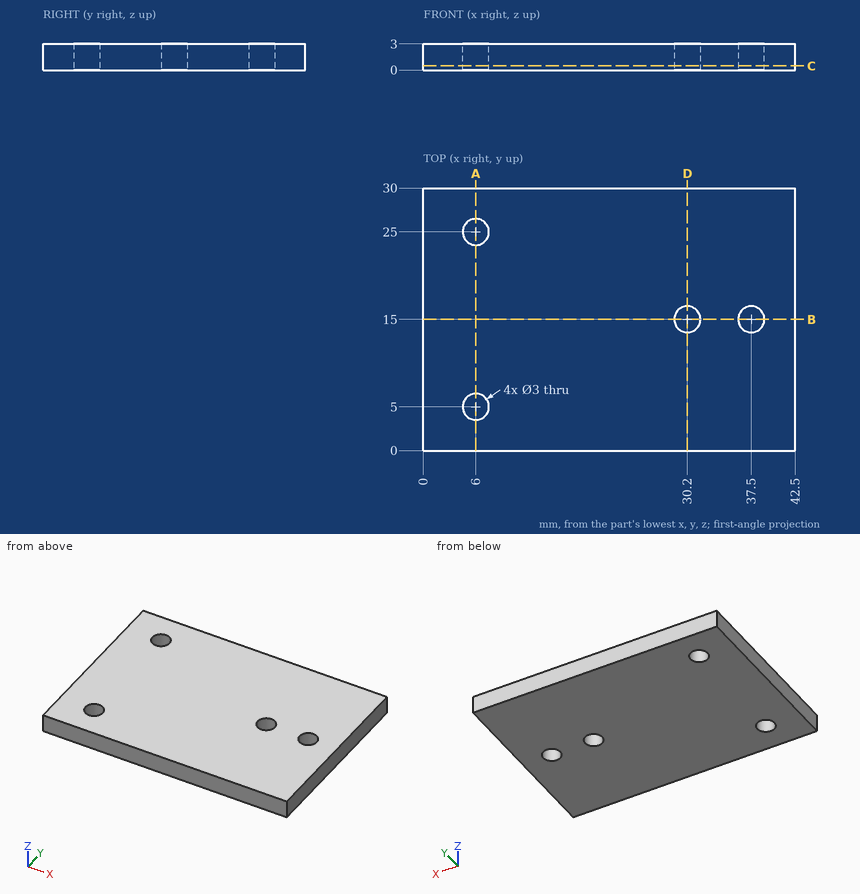
Geometry check sheet. Reference: drawing and pictorial views, mm from the part's lowest x, y, z. Round coordinates to 2 decimals unless told otherwise and drop trailing zeros. Write each loop counter-clockwise with the first axis right and the second up, starting at its lowest first coordinate (ties: lowest second). Pieces come first, ordered by that corner, then holes.
1. Gauge pin test, flat end, axial feed: P1, Ø1.8, axis at x = 6, y = 5, coming from the -Z side. Record the tip position at first contact, or that the pin passes through.
2. Section check D-D on x = 30.2. Enter the section's corners in (y, z), plus the area to 3 significant figures.
3. Section check B-B on y = 15. Enter the section's corners in (x, z).
4. Section check A-A on x = 6. Enter the section's corners in (y, z).
5. Scan lines: L1, parallel to Y at x = 6, z = 1.6; L2, parallel to Y at x = 30.2, z = 2.1; L3, parallel to X at y = 5, z = 1.75. Record each from-to range of solid material in increasing order.
6. Section check C-C on z = 0.5. Enter the section's corners in (x, y).
Answer:
1. P1: passes through
2. outline: (0, 0) - (13.5, 0) - (13.5, 3) - (0, 3) - close; (16.5, 0) - (30, 0) - (30, 3) - (16.5, 3) - close
2. area: 81.0 mm2
3. outline: (0, 0) - (28.7, 0) - (28.7, 3) - (0, 3) - close; (31.7, 0) - (36, 0) - (36, 3) - (31.7, 3) - close; (39, 0) - (42.5, 0) - (42.5, 3) - (39, 3) - close
4. outline: (0, 0) - (3.5, 0) - (3.5, 3) - (0, 3) - close; (6.5, 0) - (23.5, 0) - (23.5, 3) - (6.5, 3) - close; (26.5, 0) - (30, 0) - (30, 3) - (26.5, 3) - close
5. L1: y = 0 to 3.5, 6.5 to 23.5, 26.5 to 30
5. L2: y = 0 to 13.5, 16.5 to 30
5. L3: x = 0 to 4.5, 7.5 to 42.5
6. outline: (0, 0) - (42.5, 0) - (42.5, 30) - (0, 30) - close; hole circle Ø3 at (6, 5); hole circle Ø3 at (6, 25); hole circle Ø3 at (30.2, 15); hole circle Ø3 at (37.5, 15)
